from build123d import *

# Parameters (mm, degrees)
SKETCH_1_W     = 0.64
SKETCH_1_H     = 0.64
CHAMFER_1_SIZE = 0.1


with BuildPart() as part:
    # По траектории1: sweep along a path in Эскиз2
    with BuildLine(Plane.XY) as sweep_1_path:
        Line((0, 0), (0, 8.78))
        ThreePointArc((0, 8.78), (0.146446609, 9.133553391), (0.5, 9.28))
        Line((0.5, 9.28), (9.28, 9.28))
    # Эскиз1 → По траектории1 (sweep)
    with BuildSketch(Plane(origin=(0, 0, 0), x_dir=(1, 0, 0), z_dir=(0, 1, 0))):
        Rectangle(SKETCH_1_W, SKETCH_1_H)
    sweep(path=sweep_1_path.line)

    # Фаска1
    chamfer_1_edges = [part.edges().sort_by_distance(p)[0] for p in [
        (9.28, 8.96, 0),
        (9.28, 9.28, 0.32),
        (9.28, 9.6, 0),
        (9.28, 9.28, -0.32),
        (0, 0, 0.32),
        (-0.32, 0, 0),
        (0, 0, -0.32),
        (0.32, 0, 0),
    ]]
    chamfer(chamfer_1_edges, length=CHAMFER_1_SIZE)


solid = part.part
The model under review builds one solid part; all positions refer to its coordinate system, in mm. Coordinates: 2 decimals unless noted, no trailing zeros. Loops run counter-clockwise (first coordinate to the right, second up) from the corner with the lowest first, then second, coordinate; pieces in that order, holes last.
(1) Wall thickness on L1, parallel to Y at x = 2.25, z = 0; L2, parallel to X at y = 2.5, z = -0.05; L3, parallel to X at y = 9.25, z = -0.2: over which ranges is each line inside the solid? List them lowest first.
Determined:
L1: y = 8.96 to 9.6
L2: x = -0.32 to 0.32
L3: x = -0.17 to 9.28
(2) Consider section C-C, the plane y = 7.25. Give the boundary of the cut face in (x, z), plus the area to 3 significant figures.
Determined:
outline: (-0.32, -0.32) - (0.32, -0.32) - (0.32, 0.32) - (-0.32, 0.32) - close
area: 0.410 mm2
(3) Consider section B-B, the plane x = 4.5. Give the boundary of the cut face in (y, z), plus the area to 3 significant figures.
Determined:
outline: (8.96, -0.32) - (9.6, -0.32) - (9.6, 0.32) - (8.96, 0.32) - close
area: 0.410 mm2
(4) Consider section A-A, the plane z = 0. Give the boundary of the cut face in (x, y).
Determined:
outline: (-0.32, 0.1) - (-0.22, 0) - (0.22, 0) - (0.32, 0.1) - (0.32, 8.78) arc R0.18 cw to (0.5, 8.96) - (9.18, 8.96) - (9.28, 9.06) - (9.28, 9.5) - (9.18, 9.6) - (0.5, 9.6) arc R0.82 ccw to (-0.32, 8.78) - close
